```python
from build123d import *

# Parameters (mm, degrees)
F1_DEPTH = 2
F3_DEPTH = 100.001
F4_W     = 5
F4_H     = 7
F5_DEPTH = 7
F6_R     = 1.55
F7_DEPTH = 5


with BuildPart() as f1:
    # F0 (on Top) → F1 (new body)
    with BuildSketch(Plane.XY):
        Polygon((1, 3.5), (0, 1), (0, 0), (100, 0), (100, 1), (99, 3.5), (98, 1), (97, 3.5), (96, 1), (95, 3.5), (94, 1), (93, 3.5), (92, 1), (91, 3.5), (90, 1), (89, 3.5), (88, 1), (87, 3.5), (86, 1), (85, 3.5), (84, 1), (83, 3.5), (82, 1), (81, 3.5), (80, 1), (79, 3.5), (78, 1), (77, 3.5), (76, 1), (75, 3.5), (74, 1), (73, 3.5), (72, 1), (71, 3.5), (70, 1), (69, 3.5), (68, 1), (67, 3.5), (66, 1), (65, 3.5), (64, 1), (63, 3.5), (62, 1), (61, 3.5), (60, 1), (59, 3.5), (58, 1), (57, 3.5), (56, 1), (55, 3.5), (54, 1), (53, 3.5), (52, 1), (51, 3.5), (50, 1), (49, 3.5), (48, 1), (47, 3.5), (46, 1), (45, 3.5), (44, 1), (43, 3.5), (42, 1), (41, 3.5), (40, 1), (39, 3.5), (38, 1), (37, 3.5), (36, 1), (35, 3.5), (34, 1), (33, 3.5), (32, 1), (31, 3.5), (30, 1), (29, 3.5), (28, 1), (27, 3.5), (26, 1), (25, 3.5), (24, 1), (23, 3.5), (22, 1), (21, 3.5), (20, 1), (19, 3.5), (18, 1), (17, 3.5), (16, 1), (15, 3.5), (14, 1), (13, 3.5), (12, 1), (11, 3.5), (10, 1), (9, 3.5), (8, 1), (7, 3.5), (6, 1), (5, 3.5), (4, 1), (3, 3.5), (2, 1), align=None)
    extrude(amount=F1_DEPTH)

    # F2 (on Right) → F3 (intersect, through all)
    with BuildSketch(Plane.YZ):
        Polygon((0, 3.5), (0, 0), (3.5, 0), align=None)
    extrude(amount=F3_DEPTH, mode=Mode.INTERSECT)

    # F4 (on Top) → F5 (join)
    with BuildSketch(Plane.XY):
        with Locations((2.5, -3.5)):
            Rectangle(F4_W, F4_H)
        Polygon((5, -7), (0, -7), (-2, -7), (-2, -9), (5, -9), align=None)
    extrude(amount=F5_DEPTH)

    # F6 (on face) → F7 (cut, through all)
    with BuildSketch(Plane(origin=(0, 0, 0), x_dir=(0, -1, 0), z_dir=(-1, 0, 0))):
        with Locations((3.5, 3.5)):
            Circle(F6_R)
    extrude(amount=-F7_DEPTH, mode=Mode.SUBTRACT)


solid = f1.part
```
Work out the finished part from the listing and answer in its coordinate system (mm). A direction names the side the tool comes from. Round coordinates to 2 decimals unless told otherwise and drop trailing zeros. Loops run counter-clockwise (first coordinate to the right, second up) from the corner with the lowest first, then second, coordinate; pieces in that order, holes last. Notation, with made-up numbers: (73.5, -26) -> (95.5, -26) arc R17 cw to (95.5, -3) -> close; hole circle Ø11 at (43, -21). An arc over 180 degrees is marked (long way). Write each question's results on one line, items separated by ' | '. Start each with the question number.
1. A tool of negligible diameter and unlimited length cuts with its end or side. For faces 5 (the face through (5, -6, 3)), 6 (the face through (2, 0, 4)), 7 (the face through (1, -9, 3)), from which of +Z, -Z, +X, -X, +Y, -Y can it reach the whole face along a straight path? Write none if from no direction.
2. For a pull along X with two mould halves and no side action, classify faces 1 (the face through (89.6, 2, 0.8)), 2 (the face through (33.6, 2, 0.8)), 3 (the face through (99.6, 2, 0.8)), 4 (the face through (45, 2.3, 1.2)) as +X half, -X half, draft (parallel to the pull), parting line (faces both ways), or undercut.
3. Find the intervals of material crossed by probe 1 along Z at (x, y) = (2.35, -3.5); probe 2 along X at (y, z) = (-4.25, 5.25); probe 3 along Z at (x, y) = (25, 2.25), in increasing order. Write a range as from..to.
4. Given pin 1 Ø1 at (x, z) = (-1, 2) entering from +Y; pin 2 Ø3 at (y, z) = (-6, 0.5) entering from +X; pin 3 Ø1.2 at (x, y) = (35.5, 1) entering from +Z; pin 4 Ø4 at (x, y) = (57.5, 1) entering from -Z, each flat-ended and moving along its own axis, determine where each tip first touches the part or whether it passes through.
5. Section A-A (y = -3.5) is taken. Determine the outline of the cut face in (x, z), plus the area to 3 significant figures.
6. Section B-B (z = 3.5) is taken. Determine the outline of the cut face in (x, y).
Evaluation:
1) face 5: +Z, -Z, +X, -Y | face 6: +Z, +X, -X, +Y | face 7: +Z, -Z, +X, -X, -Y
2) face 1: undercut | face 2: undercut | face 3: +X half | face 4: draft
3) probe 1: z = 0..1.95, 5.05..7 | probe 2: x = 0..5 | probe 3: z = 0..1.25
4) pin 1: stops at y = -7 | pin 2: stops at x = 5 | pin 3: stops at z = 2 | pin 4: stops at z = 0
5) outline: (0, 0) -> (5, 0) -> (5, 1.95) -> (0, 1.95) -> close; (0, 5.05) -> (5, 5.05) -> (5, 7) -> (0, 7) -> close | area: 19.5 mm2
6) outline: (-2, -9) -> (5, -9) -> (5, -5.05) -> (0, -5.05) -> (0, -7) -> (-2, -7) -> close; (0, -1.95) -> (5, -1.95) -> (5, 0) -> (0, 0) -> close
